from build123d import *

# Parameters (mm, degrees)
RING_SKETCH_W        = 6
RING_SKETCH_H        = 22.65
NOTCH_30_DEPTH       = 6
NOTCH_60_DEPTH       = 6
NOTCH_210_DEPTH      = 6
NOTCH_240_DEPTH      = 6
SCREW_HOLE_SKETCH_W  = 1.65
SCREW_HOLE_SKETCH_H  = 9
SCREW_HOLES_X8_COUNT = 8


with BuildPart() as part:
    # Ring Sketch → Ring (revolve)
    with BuildSketch(Plane.XY, mode=Mode.PRIVATE) as ring_sk:
        with Locations((0, 87.675)):
            Rectangle(RING_SKETCH_W, RING_SKETCH_H)
    revolve(ring_sk.sketch.rotate(Axis((-1000, 0, 0), (1, 0, 0)), 90), axis=Axis((-1000, 0, 0), (1, 0, 0)))

    # Notch 30 Sketch → Notch 30 (cut)
    with BuildSketch(Plane(origin=(3, 0, 0), x_dir=(0, 0, -1), z_dir=(1, 0, 0))):
        Polygon((-48.794228634, 66.51408311), (-33.205771366, 75.51408311), (-42.705771366, 91.968565782), (-58.294228634, 82.968565782), align=None)
    extrude(amount=-NOTCH_30_DEPTH, mode=Mode.SUBTRACT)

    # Notch 60 Sketch → Notch 60 (cut)
    with BuildSketch(Plane(origin=(3, 0, 0), x_dir=(0, 0, -1), z_dir=(1, 0, 0))):
        Polygon((-75.51408311, 33.205771366), (-66.51408311, 48.794228634), (-82.968565782, 58.294228634), (-91.968565782, 42.705771366), align=None)
    extrude(amount=-NOTCH_60_DEPTH, mode=Mode.SUBTRACT)

    # Notch 210 Sketch → Notch 210 (cut)
    with BuildSketch(Plane(origin=(3, 0, 0), x_dir=(0, 0, -1), z_dir=(1, 0, 0))):
        Polygon((48.794228634, -66.51408311), (33.205771366, -75.51408311), (42.705771366, -91.968565782), (58.294228634, -82.968565782), align=None)
    extrude(amount=-NOTCH_210_DEPTH, mode=Mode.SUBTRACT)

    # Notch 240 Sketch → Notch 240 (cut)
    with BuildSketch(Plane(origin=(3, 0, 0), x_dir=(0, 0, -1), z_dir=(1, 0, 0))):
        Polygon((75.51408311, -33.205771366), (66.51408311, -48.794228634), (82.968565782, -58.294228634), (91.968565782, -42.705771366), align=None)
    extrude(amount=-NOTCH_240_DEPTH, mode=Mode.SUBTRACT)

    # Screw Hole Sketch → Screw Hole (revolve, cut)
    with BuildSketch(Plane.XY, mode=Mode.PRIVATE) as screw_hole_sk:
        with Locations((0.825, 95.5)):
            Rectangle(SCREW_HOLE_SKETCH_W, SCREW_HOLE_SKETCH_H)
    screw_hole = revolve(screw_hole_sk.sketch.rotate(Axis((0, 30, 0), (0, 1, 0)), 90), axis=Axis((0, 30, 0), (0, 1, 0)), mode=Mode.SUBTRACT)

    # Screw Holes x8: Screw Hole ×8 about axis
    screw_holes_x8_axis = Axis((0, 0, 0), (1, 0, 0))
    for i in range(1, SCREW_HOLES_X8_COUNT):
        add(screw_hole.rotate(screw_holes_x8_axis, i * 360 / SCREW_HOLES_X8_COUNT), mode=Mode.SUBTRACT)


solid = part.part
Design review of the part built by this model. Coordinates are the model's own, in mm. A direction names the side the tool comes from. Coordinates: 2 decimals unless noted, no trailing zeros. Loops run counter-clockwise (first coordinate to the right, second up) from the corner with the lowest first, then second, coordinate; pieces in that order, holes last. Notation, with made-up numbers: (-16, 48) - (-7, 48) arc R21 cw to (-7, 70) - close; hole circle Ø11 at (-8, -32). An arc over 180 degrees is marked (long way). Use CSV: the item, a comma, the result in double quotes. Start each with the question number.
1. Clearance check with flat-ended pins moving along their axes: pin 1 (3.5 mm diameter, centred on x = -1, z = -0.5, fed in from +Y); pin 2 (1 mm diameter, centred on x = 0, y = 0.5, fed in from +Z); pin 3 (2.5 mm diameter, centred on x = 0, z = 0, fed in from +Y); pin 4 (2 mm diameter, centred on x = 0.5, z = -7, fed in from +Y). State where each tip first meets the part, or that it passes through.
2. Add section A-A on z = -4. Give the boundary of the cut face in (x, y).
3. For faces 1 (the flat face through (0.04, -70.95, -41.11)), 2 (the flat face through (0, 73.8, 53)), 3 (the flat face through (0, -73.8, -53)), 4 (the flat face through (0.042, -52.884, -73.597)), list the 3-axis set-ups (+Z, -Z, +X, -X, +Y, -Y) from which the entire face can be reached by the end or side of a thin tool; tool diameter is ignored.
4. To check wall thickness, follow probe 1 along X at (y, z) = (0, -96.25); probe 2 along Z at (x, y) = (2.5, 70); probe 3 along Y at (x, z) = (0.5, 0). State the ranges of each line that lie inside material, in increasing order.
5. Mouldability with a two-part tool opening along Z and no side actions: class faces 5 (the cylindrical face through (0.709, 68.8, -71.187)), 6 (the flat face through (0.042, 52.884, 73.597)), 7 (the cylindrical face through (-0.496, 68.328, 66.102)) as released by +Z, released by -Z, zero draft, split by the parting line, or undercut.
6. Add section B-B on y = -15.5. Give the boundary of the cut face in (x, z).
Resolved:
1,pin 1,"y = 99"
1,pin 2,"z = 91"
1,pin 3,"y = 91"
1,pin 4,"y = 98.82"
2,outline,"(-3, -98.92) - (3, -98.92) - (3, -76.25) - (-3, -76.25) - close; (-3, 76.25) - (3, 76.25) - (3, 98.92) - (-3, 98.92) - close"
3,face 1,"+X, -X"
3,face 2,"+X, -X, +Y"
3,face 3,"+X, -X, -Y"
3,face 4,"-Z, +X, -X"
4,probe 1,"-3 to -1.65, 1.65 to 3"
4,probe 2,"-70.01 to -30.48, 30.48 to 42.76, 50.81 to 70.01"
4,probe 3,"-91 to -76.35, 76.35 to 91"
5,face 5,"split by the parting line"
5,face 6,"released by +Z"
5,face 7,"undercut"
6,outline,"(-3, -97.78) - (3, -97.78) - (3, -74.76) - (-3, -74.76) - close; (-3, 74.76) - (3, 74.76) - (3, 97.78) - (-3, 97.78) - close"
